Could you check a few things on this drawing? It's one solid part, dimensions in mm from its lowest x, y, z. Give positions to 0.01 mm unless a question says otherwise; leave off trailing zeros. Order: outer loops, then holes, each group sorted by start corner. A loop starts at its lowest first (then second) coordinate and runs counter-clockwise, first axis right, second up. Notation, with made-up numbers: (36, -4) -> (94, -4) arc R30 cw to (94, 34) -> close; hole circle Ø1 at (-1, 5). An arc over 180 degrees is marked (long way). Answer as a JSON object with one key per item and string values.
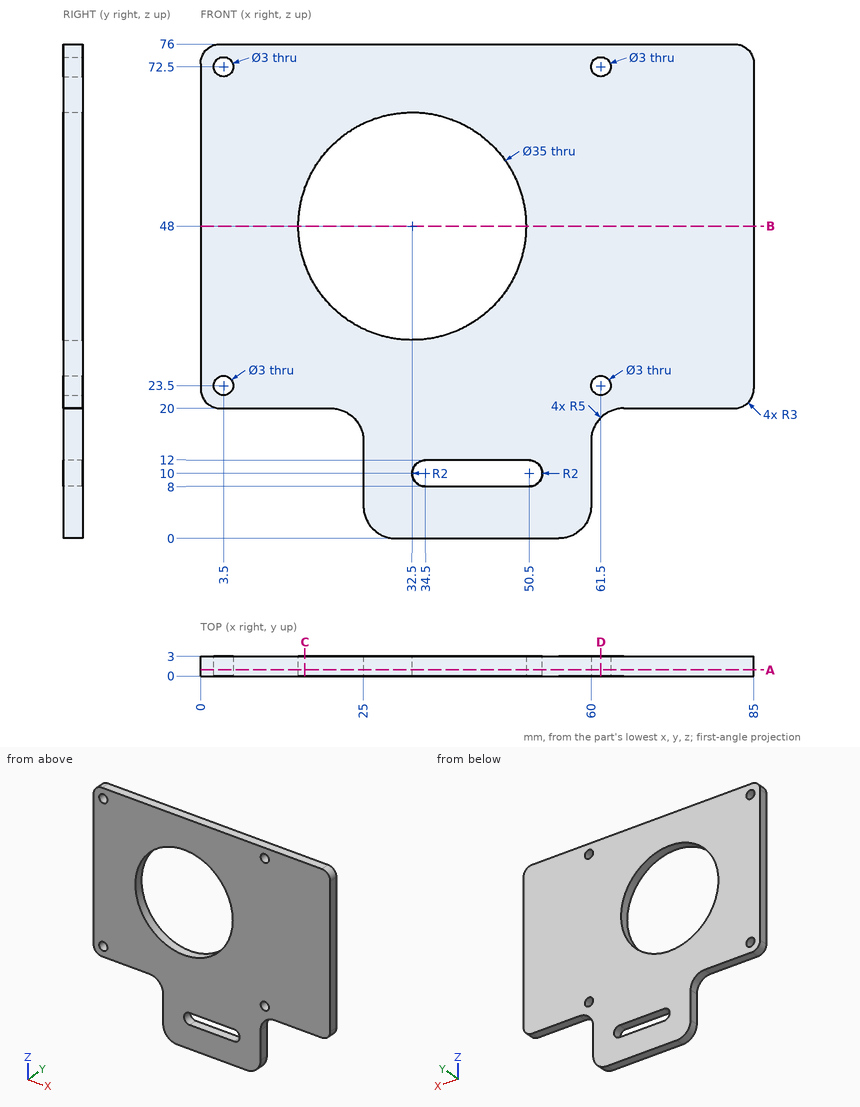
1. Will these pins go through, and if not, where does the flat tip stop? pin 1 Ø1.5 at (y, z) = (1.5, 12) entering from +X; pin 2 Ø0.9 at (x, y) = (15, 1.5) entering from -Z.
Worked answers:
{"pin 1": "x = 60", "pin 2": "z = 20"}
2. If we section it at A-A on y = 0.95: Please give me the cut outline in (x, z), then the cut area to 3 significant figures.
Worked answers:
{"outline": "(0, 23) arc R3 ccw to (3, 20) -> (20, 20) arc R5 cw to (25, 15) -> (25, 5) arc R5 ccw to (30, 0) -> (55, 0) arc R5 ccw to (60, 5) -> (60, 15) arc R5 cw to (65, 20) -> (82, 20) arc R3 ccw to (85, 23) -> (85, 73) arc R3 ccw to (82, 76) -> (3, 76) arc R3 ccw to (0, 73) -> close; hole circle Ø3 at (3.5, 23.5); hole circle Ø3 at (3.5, 72.5); hole circle Ø35 at (32.5, 48); hole (34.5, 8) -> (50.5, 8) arc R2 ccw to (50.5, 12) -> (34.5, 12) arc R2 ccw to start; hole circle Ø3 at (61.5, 23.5); hole circle Ø3 at (61.5, 72.5)", "area": "4,390 mm²"}
3. Please list where these lines run through material, in increasing order: L1, parallel to Z at x = 3.5, y = 1.65; L2, parallel to X at y = 2.3, z = 23.5; L3, parallel to X at y = 2.1, z = 48.
Worked answers:
{"L1": "20 to 22, 25 to 71, 74 to 76", "L2": "0 to 2, 5 to 60, 63 to 85", "L3": "0 to 15, 50 to 85"}
4. If we section it at B-B on z = 48: Please give me the cut outline in (x, y).
Worked answers:
{"outline": "(0, 0) -> (15, 0) -> (15, 3) -> (0, 3) -> close; (50, 0) -> (85, 0) -> (85, 3) -> (50, 3) -> close"}
5. If we section it at C-C on x = 16: Please give me the cut outline in (y, z).
Worked answers:
{"outline": "(0, 20) -> (3, 20) -> (3, 42.17) -> (0, 42.17) -> close; (0, 53.83) -> (3, 53.83) -> (3, 76) -> (0, 76) -> close"}
6. If we section it at D-D on x = 61.5: Please give me the cut outline in (y, z), then the cut area to 3 significant figures.
Worked answers:
{"outline": "(0, 18.57) -> (3, 18.57) -> (3, 22) -> (0, 22) -> close; (0, 25) -> (3, 25) -> (3, 71) -> (0, 71) -> close; (0, 74) -> (3, 74) -> (3, 76) -> (0, 76) -> close", "area": "154 mm²"}
